```python
from build123d import *

# Parameters (mm, degrees)
PAD_DEPTH          = 30
PAD001_DEPTH       = 15
POLARPATTERN_COUNT = 4


with BuildPart() as part:
    # Sketch (on XY_Plane of Origin) → Pad (new body)
    with BuildSketch(Plane.XY):
        with BuildLine():
            ThreePointArc((244.764719, -18.871714), (167.483272, 24.840105), (80, 40))
            ThreePointArc((80, 40), (40, 0), (80, -40))
            ThreePointArc((194.067882, -80.75734), (140.565342, -50.495312), (80, -40))
            ThreePointArc((194.067882, -80.75734), (250.359114, -75.162945), (244.764719, -18.871714))
        make_face()
        with BuildLine():
            ThreePointArc((206.742091, -65.285934), (147.294824, -31.661457), (80, -20))
            ThreePointArc((80, 20), (60, 0), (80, -20))
            ThreePointArc((232.09051, -34.34312), (160.753789, 6.006251), (80, 20))
            ThreePointArc((206.742091, -65.285934), (234.887707, -62.488736), (232.09051, -34.34312))
        make_face(mode=Mode.SUBTRACT)
    extrude(amount=PAD_DEPTH)

    # Sketch001 (on XY_Plane of Origin) → Pad001 (join)
    with BuildSketch(Plane.XY):
        with BuildLine():
            ThreePointArc((14.849242, -14.849242), (21, 0), (14.849242, 14.849242))
            Line((14.849242, 14.849242), (45.670006, 45.670006))
            ThreePointArc((45.670006, 45.670006), (56.892253, 38.894945), (70, 38.729833))
            ThreePointArc((70, 38.729833), (40, 0), (70, -38.729833))
            ThreePointArc((70, -38.729833), (56.892253, -38.894945), (45.670006, -45.670006))
            Line((45.670006, -45.670006), (14.849242, -14.849242))
        make_face()
    extrude(amount=PAD001_DEPTH)

    # PolarPattern: part ×4 about axis
    polarpattern_axis = Axis((0, 0, 0), (0, 0, 1))


with BuildPart() as part_1:
    add(part.part)
    for i in range(1, POLARPATTERN_COUNT):
        add(part.part.rotate(polarpattern_axis, i * 360 / POLARPATTERN_COUNT))


solid = part_1.part
```
Build history of the part. All positions in model axes, mm. A direction names the side the tool comes from. Give positions to 0.01 mm unless a question says otherwise; leave off trailing zeros. Loops run counter-clockwise (first coordinate to the right, second up) from the corner with the lowest first, then second, coordinate; pieces in that order, holes last.
1) Probe line 1 along Y through (x, z) = (-84, 21.25); line 2 along Y through (x, z) = (0, 7.5); line 3 along Y through (x, z) = (-72, 3.5). List the from-to ranges inside material, lowest first.
Values follow:
line 1: y = -240.19 to -198.65, -39.97 to -19.97, 20.04 to 40.04
line 2: y = -218.56 to -175.92, -60 to -21, 21 to 60, 175.92 to 218.56
line 3: y = -252.7 to -182.45, -39.19 to -18.33, 18.33 to 39.19
2) Band-saw the part on B-B on y = 154. List the corners of the cut face in (x, z), then the cut area to 3 significant figures.
Values follow:
outline: (-29.25, 0) - (-8.31, 0) - (-8.31, 30) - (-29.25, 30) - close; (34.19, 0) - (55.91, 0) - (55.91, 30) - (34.19, 30) - close
area: 1,280 mm2
3) Band-saw the part on A-A on x = 148. List the corners of the cut face in (y, z).
Values follow:
outline: (-53.34, 0) - (-31.91, 0) - (-31.91, 30) - (-53.34, 30) - close; (10.17, 0) - (30.95, 0) - (30.95, 30) - (10.17, 30) - close
4) Two-plate mould, pull along Y, no slides. Class faces 1 (the face through (-141.38, 50.79, 14.79)), 2 (the face through (-75.84, -249.79, 14.79)), 3 (the face through (141.38, -50.79, 14.79)): released by +Y, released by -Y, zero draft, split by the parting line, or undercut.
Values follow:
face 1: released by +Y
face 2: undercut
face 3: released by -Y
5) Drop flat-ended pins along their axis: P1, Ø6, axis at y = 180, z = 25.5, coming from the +X side; P2, Ø10, axis at y = -80.5, z = 23.5, coming from the +X side; P3, Ø4, axis at y = -146, z = 13, coming from the -X side. Give the stop position or say it passes through.
Values follow:
P1: stops at x = 72.38
P2: stops at x = 250.08
P3: stops at x = -53.34
6) Band-saw the part on C-C on y = 0. List the corners of the cut face in (x, z), then the cut area to 3 significant figures.
Values follow:
outline: (-218.56, 0) - (-175.92, 0) - (-175.92, 30) - (-218.56, 30) - close; (-60, 0) - (-21, 0) - (-21, 15) - (-40, 15) - (-40, 30) - (-60, 30) - close; (21, 0) - (60, 0) - (60, 30) - (40, 30) - (40, 15) - (21, 15) - close; (175.92, 0) - (218.56, 0) - (218.56, 30) - (175.92, 30) - close
area: 4,330 mm2
7) 3-axis set-ups, long thin cutter, end or side, ignore diameter. For faces 4 (the face through (-57.069, 38.845, 7.395)), 5 (the face through (56.712, 38.947, 7.395)), 6 (the face through (-40.01, -0.88, 21.46)): which of +Z, -Z, +X, -X, +Y, -Y reach the whole face in a straight line?
Values follow:
face 4: +Z, -Z, +Y
face 5: +Z, -Z
face 6: +Z
